Verification items for the finished model (mm, model axes). Give positions to 0.01 mm unless a question says otherwise; leave off trailing zeros. Write each loop counter-clockwise with the first axis right and the second up, starting at its lowest first coordinate (ties: lowest second). Pieces come first, ordered by that corner, then holes. Notation, with made-up numbers: (-30, 82.5) - (28, 82.5) arc R21 ccw to (28, 109.5) - close; hole circle Ø1 at (35, 12.25). An arc over 180 degrees is marked (long way). Put each result on its own line as item: value.
from build123d import *

# Parameters (mm, degrees)
REVOLVE1_ANGLE                 = 90
BOSS_EXTRUDE2_DEPTH            = 22.5
CUT_EXTRUDE1_DEPTH             = 74.549310272
MIRROR3_START                  = -2.736132077
MIRROR3_DEPTH                  = 5
MIRROR3_START_2                = 2.263867923
MIRROR3_2_DEPTH                = 20.236132077
MIRROR3_3_DEPTH                = 1
MIRROR3_START_3                = 1.263867923
MIRROR3_4_DEPTH                = 1
MIRROR4_START                  = -2.736132077
MIRROR4_DEPTH                  = 5
MIRROR4_START_2                = 2.263867923
MIRROR4_2_DEPTH                = 20.236132077
MIRROR4_3_DEPTH                = 1
MIRROR4_START_3                = 1.263867923
MIRROR4_4_DEPTH                = 1
SKETCH7_R                      = 3.35
CUT_EXTRUDE2_DEPTH             = 20
FILLET9_R                      = 0.5
CUT_EXTRUDE3_REACH             = 76.204
SKETCH8_R                      = 1.5
CUT_EXTRUDE3_DIRECTION_2_REACH = 76.204


# Read off the part's stored shape, not the designer's step: Mirror3, Mirror4
with BuildPart() as part:
    # Sketch1 → Revolve1 (revolve)
    with BuildSketch(Plane.XY):
        Polygon((0, 2.263867923), (0, -2.736132077), (50, -2.736132077), (50, -1.736132077), (49.75, -1.736132077), (49.75, 1.263867923), (50, 1.263867923), (50, 2.263867923), align=None)
    revolve(axis=Axis((0, 2.263867923, 0), (0, -1, 0)), revolution_arc=REVOLVE1_ANGLE)

    # Sketch2 → Boss-Extrude2 (add)
    with BuildSketch(Plane(origin=(0, 0, 0), x_dir=(1, 0, 0), z_dir=(0, 1, 0))):
        with BuildLine():
            Line((0, 0), (6, 0))
            ThreePointArc((6, 0), (4.242640687, -4.242640687), (0, -6))
            Line((0, -6), (0, 0))
        make_face()
    extrude(amount=BOSS_EXTRUDE2_DEPTH)

    # Sketch6 → Cut-Extrude1 (cut, through all)
    with BuildSketch(Plane(origin=(0, 2.263867923, 0), x_dir=(1, 0, 0), z_dir=(0, 1, 0))):
        with BuildLine():
            Line((2, -5.656854249), (2, -44.955533586))
            ThreePointArc((2, -44.955533586), (31.819805153, -31.819805153), (44.955533586, -2))
            Line((44.955533586, -2), (5.656854249, -2))
            ThreePointArc((5.656854249, -2), (4.242640687, -4.242640687), (2, -5.656854249))
        make_face()
    extrude(amount=-CUT_EXTRUDE1_DEPTH, mode=Mode.SUBTRACT)

    # Mirror3 outline → Mirror3 (add)
    with BuildSketch(Plane(origin=(0, 0, 0), x_dir=(1, 0, 0), z_dir=(0, 1, 0)).offset(MIRROR3_START)):
        with BuildLine():
            ThreePointArc((49.75, 0), (35.178562364, 35.178562364), (0, 49.75))
            Line((0, 49.75), (0, 0))
            Line((0, 0), (49.75, 0))
        make_face()
        with BuildLine():
            Line((44.955533586, 2), (5.656854249, 2))
            ThreePointArc((5.656854249, 2), (4.242640687, 4.242640687), (2, 5.656854249))
            Line((2, 5.656854249), (2, 44.955533586))
            ThreePointArc((2, 44.955533586), (31.819805153, 31.819805153), (44.955533586, 2))
        make_face(mode=Mode.SUBTRACT)
    extrude(amount=MIRROR3_DEPTH)

    # Mirror3 2 outline → Mirror3 2 (add)
    with BuildSketch(Plane(origin=(0, 0, 0), x_dir=(1, 0, 0), z_dir=(0, 1, 0)).offset(MIRROR3_START_2)):
        with BuildLine():
            Line((0, 0), (6, 0))
            ThreePointArc((6, 0), (4.242640687, 4.242640687), (0, 6))
            Line((0, 6), (0, 0))
        make_face()
    extrude(amount=MIRROR3_2_DEPTH)

    # Mirror3 3 outline → Mirror3 3 (add)
    with BuildSketch(Plane(origin=(0, 0, 0), x_dir=(1, 0, 0), z_dir=(0, 1, 0)).offset(MIRROR3_START)):
        with BuildLine():
            Line((49.75, 0), (50, 0))
            ThreePointArc((50, 0), (35.355339059, 35.355339059), (0, 50))
            Line((0, 50), (0, 49.75))
            ThreePointArc((0, 49.75), (35.178562364, 35.178562364), (49.75, 0))
        make_face()
    extrude(amount=MIRROR3_3_DEPTH)

    # Mirror3 4 outline → Mirror3 4 (add)
    with BuildSketch(Plane(origin=(0, 0, 0), x_dir=(1, 0, 0), z_dir=(0, 1, 0)).offset(MIRROR3_START_3)):
        with BuildLine():
            Line((49.75, 0), (50, 0))
            ThreePointArc((50, 0), (35.355339059, 35.355339059), (0, 50))
            Line((0, 50), (0, 49.75))
            ThreePointArc((0, 49.75), (35.178562364, 35.178562364), (49.75, 0))
        make_face()
    extrude(amount=MIRROR3_4_DEPTH)

    # Mirror4 outline → Mirror4 (add)
    with BuildSketch(Plane(origin=(0, 0, 0), x_dir=(1, 0, 0), z_dir=(0, 1, 0)).offset(MIRROR4_START)):
        with BuildLine():
            ThreePointArc((0, 49.75), (-49.75, 0), (0, -49.75))
            Line((0, -49.75), (0, 49.75))
        make_face()
        with BuildLine():
            Line((-2, 44.955533586), (-2, 5.656854249))
            ThreePointArc((-2, 5.656854249), (-4.242640687, 4.242640687), (-5.656854249, 2))
            Line((-5.656854249, 2), (-44.955533586, 2))
            ThreePointArc((-44.955533586, 2), (-31.819805153, 31.819805153), (-2, 44.955533586))
        make_face(mode=Mode.SUBTRACT)
        with BuildLine():
            Line((-44.955533586, -2), (-5.656854249, -2))
            ThreePointArc((-5.656854249, -2), (-4.242640687, -4.242640687), (-2, -5.656854249))
            Line((-2, -5.656854249), (-2, -44.955533586))
            ThreePointArc((-2, -44.955533586), (-31.819805153, -31.819805153), (-44.955533586, -2))
        make_face(mode=Mode.SUBTRACT)
    extrude(amount=MIRROR4_DEPTH)

    # Mirror4 2 outline → Mirror4 2 (add)
    with BuildSketch(Plane(origin=(0, 0, 0), x_dir=(1, 0, 0), z_dir=(0, 1, 0)).offset(MIRROR4_START_2)):
        with BuildLine():
            Line((0, -6), (0, 6))
            ThreePointArc((0, 6), (-6, 0), (0, -6))
        make_face()
    extrude(amount=MIRROR4_2_DEPTH)

    # Mirror4 3 outline → Mirror4 3 (add)
    with BuildSketch(Plane(origin=(0, 0, 0), x_dir=(1, 0, 0), z_dir=(0, 1, 0)).offset(MIRROR4_START)):
        with BuildLine():
            Line((0, 49.75), (0, 50))
            ThreePointArc((0, 50), (-50, 0), (0, -50))
            Line((0, -50), (0, -49.75))
            ThreePointArc((0, -49.75), (-49.75, 0), (0, 49.75))
        make_face()
    extrude(amount=MIRROR4_3_DEPTH)

    # Mirror4 4 outline → Mirror4 4 (add)
    with BuildSketch(Plane(origin=(0, 0, 0), x_dir=(1, 0, 0), z_dir=(0, 1, 0)).offset(MIRROR4_START_3)):
        with BuildLine():
            Line((0, 49.75), (0, 50))
            ThreePointArc((0, 50), (-50, 0), (0, -50))
            Line((0, -50), (0, -49.75))
            ThreePointArc((0, -49.75), (-49.75, 0), (0, 49.75))
        make_face()
    extrude(amount=MIRROR4_4_DEPTH)

    # Sketch7 → Cut-Extrude2 (cut)
    with BuildSketch(Plane(origin=(0, 22.5, 0), x_dir=(1, 0, 0), z_dir=(0, 1, 0))):
        with Locations(Location((0, 0, 0), (0, 0, 270))):
            Circle(SKETCH7_R)
    extrude(amount=-CUT_EXTRUDE2_DEPTH, mode=Mode.SUBTRACT)

    # Fillet9
    # the kernel refuses this fillet: 0.5 mm, written as the material it adds along each edge
    with BuildSketch(Plane(origin=(0, 1.263867923, 0), x_dir=(0, 0, 1), z_dir=(1, 0, 0))) as fillet9_piece_1:
        with BuildLine():
            CenterArc((50.25, 0.433012702), FILLET9_R, 180, 60)
            Line((50, 0), (49.995, -0.008660254))
            ThreePointArc((49.995, -0.008660254), (49.875, -0.01), (49.75, -0.01))
            Line((49.75, -0.01), (49.74, 0))
            Line((49.74, 0), (49.74, 0.433012702))
            Line((49.74, 0.433012702), (49.75, 0.433012702))
        make_face()
    revolve(axis=Axis((0, 1.263867923, 0), (0, -1, 0)), revolution_arc=180)
    with BuildSketch(Plane(origin=(0, -1.736132077, 0), x_dir=(0, 0, 1), z_dir=(1, 0, 0))) as fillet9_piece_2:
        with BuildLine():
            CenterArc((50.25, -0.433012702), FILLET9_R, 120, 60)
            Line((49.75, -0.433012702), (49.74, -0.433012702))
            Line((49.74, -0.433012702), (49.74, 0))
            Line((49.74, 0), (49.75, 0.01))
            ThreePointArc((49.75, 0.01), (49.875, 0.01), (49.995, 0.008660254))
            Line((49.995, 0.008660254), (50, 0))
        make_face()
    revolve(axis=Axis((0, -1.736132077, 0), (0, -1, 0)), revolution_arc=180)
    with BuildSketch(Plane(origin=(0, -1.736132077, 0), x_dir=(1, 0, 0), z_dir=(0, 0, -1))) as fillet9_piece_3:
        with BuildLine():
            CenterArc((50.25, -0.433012702), FILLET9_R, 120, 60)
            Line((49.75, -0.433012702), (49.74, -0.433012702))
            Line((49.74, -0.433012702), (49.74, 0))
            Line((49.74, 0), (49.75, 0.01))
            ThreePointArc((49.75, 0.01), (49.875, 0.01), (49.995, 0.008660254))
            Line((49.995, 0.008660254), (50, 0))
        make_face()
    revolve(axis=Axis((0, -1.736132077, 0), (0, -1, 0)), revolution_arc=90)
    with BuildSketch(Plane(origin=(0, -1.736132077, 0), x_dir=(2.109490694905436e-12, 0, -1.0), z_dir=(-1.0, 0, -2.109490694905436e-12))) as fillet9_piece_4:
        with BuildLine():
            CenterArc((50.25, -0.433012702), FILLET9_R, 120, 60)
            Line((49.75, -0.433012702), (49.74, -0.433012702))
            Line((49.74, -0.433012702), (49.74, 0))
            Line((49.74, 0), (49.75, 0.01))
            ThreePointArc((49.75, 0.01), (49.875, 0.01), (49.995, 0.008660254))
            Line((49.995, 0.008660254), (50, 0))
        make_face()
    revolve(axis=Axis((0, -1.736132077, 0), (0, -1, 0)), revolution_arc=90)
    with BuildSketch(Plane(origin=(0, 1.263867923, 0), x_dir=(1, 0, 0), z_dir=(0, 0, -1))) as fillet9_piece_5:
        with BuildLine():
            CenterArc((50.25, 0.433012702), FILLET9_R, 180, 60)
            Line((50, 0), (49.995, -0.008660254))
            ThreePointArc((49.995, -0.008660254), (49.875, -0.01), (49.75, -0.01))
            Line((49.75, -0.01), (49.74, 0))
            Line((49.74, 0), (49.74, 0.433012702))
            Line((49.74, 0.433012702), (49.75, 0.433012702))
        make_face()
    revolve(axis=Axis((0, 1.263867923, 0), (0, -1, 0)), revolution_arc=90)
    with BuildSketch(Plane(origin=(0, 1.263867923, 0), x_dir=(2.109490694905436e-12, 0, -1.0), z_dir=(-1.0, 0, -2.109490694905436e-12))) as fillet9_piece_6:
        with BuildLine():
            CenterArc((50.25, 0.433012702), FILLET9_R, 180, 60)
            Line((50, 0), (49.995, -0.008660254))
            ThreePointArc((49.995, -0.008660254), (49.875, -0.01), (49.75, -0.01))
            Line((49.75, -0.01), (49.74, 0))
            Line((49.74, 0), (49.74, 0.433012702))
            Line((49.74, 0.433012702), (49.75, 0.433012702))
        make_face()
    revolve(axis=Axis((0, 1.263867923, 0), (0, -1, 0)), revolution_arc=90)

    # Sketch8 → Cut-Extrude3 (cut, up to next)
    with BuildSketch(Plane.XY, mode=Mode.PRIVATE) as cut_extrude3_sk1:
        with Locations((0, 12.5)):
            Circle(SKETCH8_R)
    cut_extrude3_tool1 = extrude(cut_extrude3_sk1.sketch, amount=-CUT_EXTRUDE3_REACH, mode=Mode.PRIVATE) & part.part
    add(cut_extrude3_tool1.solids().sort_by_distance((0, 12.5, 0))[0], mode=Mode.SUBTRACT)

    # Sketch8 → Cut-Extrude3 direction 2 (cut, up to next)
    with BuildSketch(Plane.XY, mode=Mode.PRIVATE) as cut_extrude3_direction_2_sk1:
        with Locations((0, 12.5)):
            Circle(SKETCH8_R)
    cut_extrude3_direction_2_tool1 = extrude(cut_extrude3_direction_2_sk1.sketch, amount=CUT_EXTRUDE3_DIRECTION_2_REACH, mode=Mode.PRIVATE) & part.part
    add(cut_extrude3_direction_2_tool1.solids().sort_by_distance((0, 12.5, 0))[0], mode=Mode.SUBTRACT)


solid = part.part
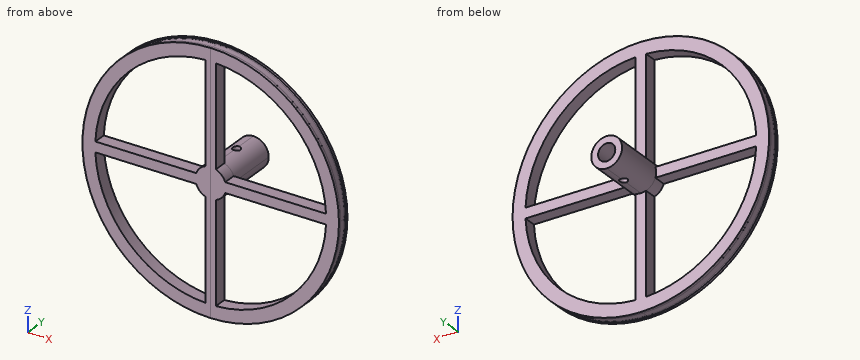
Q1. Go/stop test with flat-tipped pins: pin 1 Ø6 at (x, y) = (24, 1.5) entering from -Z; pin 2 Ø4 at (x, y) = (-26, -1.5) entering from -Z; pin 3 Ø5.5 at (x, y) = (-16, 1) entering from +Z; pin 4 Ø7.5 at (x, z) = (0, -0.5) entering from +Y. Record where each tip stops, or that it passes through.
Answers follow:
pin 1: stops at z = -45.38
pin 2: stops at z = -43.86
pin 3: stops at z = 48.21
pin 4: stops at y = 22.5
Q2. Section check C-C, the plane z = -36.5. Give the number of separate pieces and of enclosed holes in the cut face, plus the area to 3 significant figures.
Answers follow:
separate pieces: 3
enclosed holes: 0
area: 96.5 mm2
Q3. Section check A-A, the plane y = 6.5. Record the cut outline in (x, z), plus the area to 3 significant figures.
Answers follow:
outline: circle Ø12 at (0, 0); hole circle Ø6.7 at (0, 0)
area: 77.8 mm2
Q4. Section check B-B, the plane y = 12.5. Record the cut outline in (x, z), plus the area to 3 significant figures.
Answers follow:
outline: (-1.5, -5.81) - (-1.5, -3) arc R3.35 cw to (-1.5, 3) - (-1.5, 5.81) arc R6 ccw to start; (1.5, -5.81) arc R6 ccw to (1.5, 5.81) - (1.5, 3) arc R3.35 cw to (1.5, -3) - close
area: 61.6 mm2
Q5. Scan lines: line 1 along Z through (x, y) = (0, 15.25); line 2 along X through (y, z) = (-0.5, -37); line 3 along Z through (x, y) = (-10.5, -1.5). Record each from-to range of solid material in increasing order.
Answers follow:
line 1: z = -6 to -3.35, 3.35 to 6
line 2: x = -33.26 to -25.61, -2 to 2, 25.61 to 33.26
line 3: z = -48.67 to -43.76, -2 to 2, 43.76 to 48.67
